Build history of the part. All positions in model axes, mm. A direction names the side the tool comes from. Give positions to 0.01 mm unless a question says otherwise; leave off trailing zeros. Order: outer loops, then holes, each group sorted by start corner. A loop starts at its lowest first (then second) coordinate and runs counter-clockwise, first axis right, second up. Notation, with made-up numbers: (41.25, -6.5) - (74.25, -6.5) arc R10 cw to (74.25, -1.5) - close; hole circle Ø2 at (70.5, -9). An arc over 180 degrees is marked (long way). Use a Markdown table: item, result. Add a question column.
(1) Slice it at B-B (z = 6.75). Write the cut outline in (x, y), then the cut area to 3 significant figures.
(2) Which spindle directions (+Z, -Z, +X, -X, +Y, -Y) get a long thin tool onto all of the face, cutting with end or side? Do faces 1 (the face through (-3, 3, 7)), 2 (the face through (-4, 28, 10)), 3 (the face through (0, 36, 0)), 4 (the face through (-6, 1, 6)), 5 (the face through (0, 35, 4)). Say none if no direction does.
(3) Flat gauge pins, fed straight in: pin 1 (1.5 mm diameter, centred on y = 95.5, z = 4, fed in from +X); pin 2 (5.5 mm diameter, centred on y = -9.5, z = 6.5, fed in from -X). Where does each tip first touch, or does it go through?
(4) Mould opens along X. For faces 6 (the face through (3, 0, 7)), 7 (the face through (-0.1, -100, 3.8)), 8 (the face through (0.309, 118.386, 7.042)), 9 (the face through (6, -1, 6)) say: +X half, -X half, draft (parallel to the pull), parting line (faces both ways), or undercut.
(5) Slice it at A-A (y = 55). Write the cut outline in (x, z), then the cut area to 3 significant figures.
(6) Wall check: line 1 (X direction, y = 52, z = 8); line 2 (Y direction, x = 0, z = 5.45); line 3 (Z direction, x = 0.5, y = -60). Give the ranges that are in metal, low to high.
from build123d import *

# Parameters (mm, degrees)
F1_DEPTH = 10
F3_DEPTH = 6
F4_R     = 3


with BuildPart() as f1:
    # F0 (on Top) → F1 (new body)
    with BuildSketch(Plane.XY):
        with BuildLine():
            ThreePointArc((12, 110.3923048454), (-6, 120.7846096908), (-6, 100))
            Line((-6, 100), (6, 100))
            ThreePointArc((6, 100), (10.3923048454, 104.3923048454), (12, 110.3923048454))
        make_face()
        with BuildLine():
            ThreePointArc((6, 100), (0, 98.3923048454), (-6, 100))
            Line((-6, 100), (-6, -100))
            Line((-6, -100), (6, -100))
            Line((6, -100), (6, 100))
        make_face()
        with BuildLine():
            Line((6, 100), (-6, 100))
            ThreePointArc((-6, 100), (0, 98.3923048454), (6, 100))
        make_face()
    extrude(amount=F1_DEPTH)

    # F2 (on face) → F3 (cut)
    with BuildSketch(Plane.XY.offset(10)):
        with BuildLine():
            Line((3, -100), (3, 102.9761063583))
            ThreePointArc((3, 102.9761063583), (0, 118.3923048454), (-3, 102.9761063583))
            Line((-3, 102.9761063583), (-3, -100))
            Line((-3, -100), (3, -100))
        make_face()
    extrude(amount=-F3_DEPTH, mode=Mode.SUBTRACT)

    # F4
    f4_edges = [f1.edges().sort_by_distance(p)[0] for p in [
        (6, 0, 0),
        (0, 122.392305, 0),
        (-6, 0, 0),
    ]]
    fillet(f4_edges, radius=F4_R)


solid = f1.part
Solution:
| question | item | result |
|---|---|---|
| 1 | outline | (-6, -100) - (-3, -100) - (-3, 102.98) arc R8 cw (long way) to (3, 102.98) - (3, -100) - (6, -100) - (6, 100) arc R12 ccw (long way) to (-6, 100) - close |
| 1 | area | 1,420 mm2 |
| 2 | face 1 | +Z, -Y |
| 2 | face 2 | +Z, +X, -X, +Y, -Y |
| 2 | face 3 | -Z, +X, -X, +Y, -Y |
| 2 | face 4 | +Z, -Z, -X, -Y |
| 2 | face 5 | +Z |
| 3 | pin 1 | x = 6 |
| 3 | pin 2 | x = -6 |
| 4 | face 6 | undercut |
| 4 | face 7 | draft |
| 4 | face 8 | undercut |
| 4 | face 9 | +X half |
| 5 | outline | (-6, 3) arc R3 ccw to (-3, 0) - (3, 0) arc R3 ccw to (6, 3) - (6, 10) - (3, 10) - (3, 4) - (-3, 4) - (-3, 10) - (-6, 10) - close |
| 5 | area | 80.1 mm2 |
| 6 | line 1 | -6 to -3, 3 to 6 |
| 6 | line 2 | 118.39 to 122.39 |
| 6 | line 3 | 0 to 4 |
